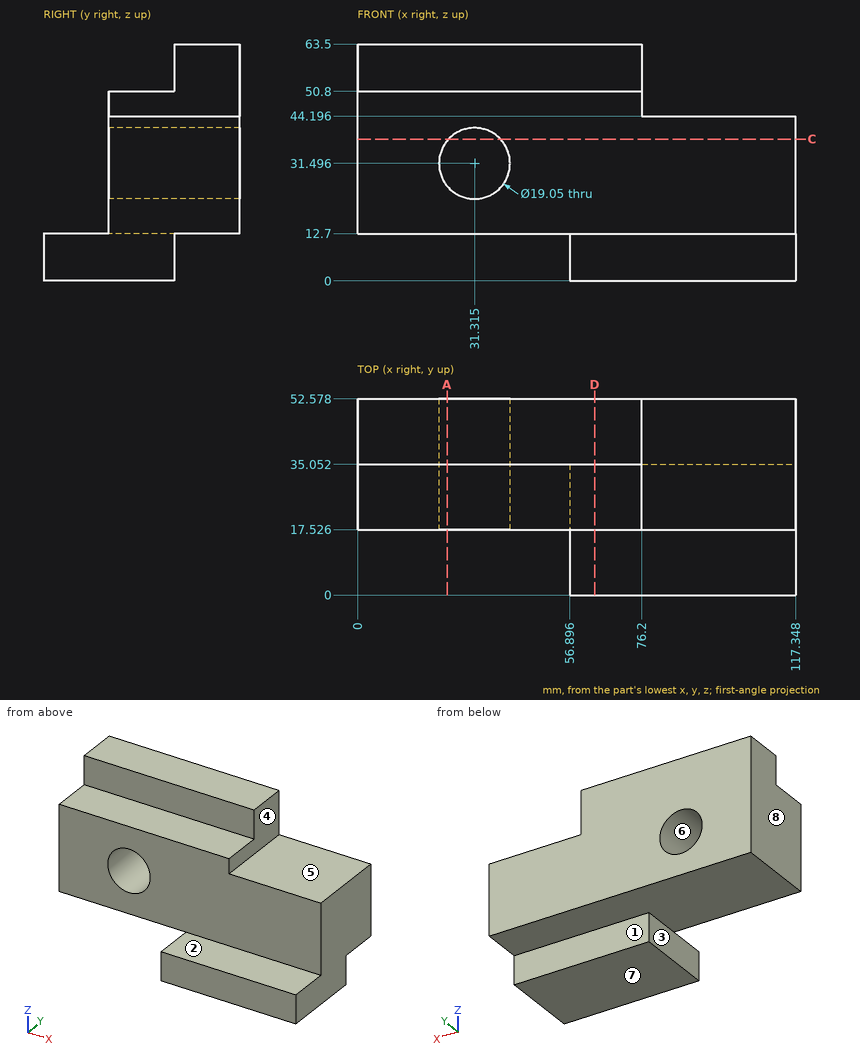
Input: dimensioned drawing with shaded views. Units: mm. Origin: part minimum x, y, z. A direction names the side the tool comes from. Round coordinates to 2 decimals unless told otherwise and drop trailing zeros. Loops run counter-clockwise (first coordinate to the right, second up) from the corner with the lowest first, then second, coordinate; pieces in that order, holes last. Notation, with made-up numbers: (-2.75, -33.5) -> (21.25, -33.5) arc R27 cw to (21.25, 1.5) -> close; hole circle Ø3 at (45.25, 32). An arc over 180 degrees is marked (long way). Answer as a JSON object with one key per item and string values. Group by question number.
1) Reachability of the marked faces 1, 2, 3 and 4 from +Z, -Z, +X, -X, +Y, -Y: full face, straight path, thin tool, end or side. Return the list, or none.
2) Section query D-D on x = 63.5. Output: boundary loops of the cut face in (y, z).
3) Section query A-A on x = 24. Output: boundary loops of the cut face in (y, z).
4) Draft query along Z for the marked faces 5, 6, 7 and 8. Return one class per face: +Z half, -Z half, draft (parallel to the pull), parting line (faces both ways), or undercut.
5) Ray query, L1, parallel to Y at x = 43, z = 58.5; L2, parallel to Z at x = 90.5, y = 27.5; L3, parallel to Z at x = 100, y = 17. Return the intervals inside material, ascending.
6) Section query C-C on z = 38. Output: boundary loops of the cut face in (x, y), plus the area to 3 significant figures.
7) Pin query (flat end, axial travel): pin 1 (4 mm diameter, centred on x = 86.5, z = 4, fed in from +Y); pin 2 (14 mm diameter, centred on y = 24.5, z = 5.5, fed in from -X); pin 3 (1 mm diameter, centred on x = 29, z = 55.5, fed in from -Y); pin 4 (15 mm diameter, centred on x = 31.32, z = 31.5, fed in from -Y). Return the tip coordinate at first contact, or that it passes through.
Reply:
{
 "1": {"face 1": "-Z, +X, -X, +Y", "face 2": "+Z, +X, -X, -Y", "face 3": "-Z, -X, +Y, -Y", "face 4": "+Z, +X, +Y, -Y"},
 "2": {"outline": "(0, 0) -> (35.05, 0) -> (35.05, 12.7) -> (52.58, 12.7) -> (52.58, 63.5) -> (35.05, 63.5) -> (35.05, 50.8) -> (17.53, 50.8) -> (17.53, 12.7) -> (0, 12.7) -> close"},
 "3": {"outline": "(17.53, 12.7) -> (52.58, 12.7) -> (52.58, 25.4) -> (17.53, 25.4) -> close; (17.53, 37.6) -> (52.58, 37.6) -> (52.58, 63.5) -> (35.05, 63.5) -> (35.05, 50.8) -> (17.53, 50.8) -> close"},
 "4": {"face 5": "+Z half", "face 6": "undercut", "face 7": "-Z half", "face 8": "draft"},
 "5": {"L1": "y = 35.05 to 52.58", "L2": "z = 0 to 44.2", "L3": "z = 0 to 12.7"},
 "6": {"outline": "(0, 17.53) -> (24.36, 17.53) -> (24.36, 52.58) -> (0, 52.58) -> close; (38.27, 17.53) -> (117.35, 17.53) -> (117.35, 52.58) -> (38.27, 52.58) -> close", "area": "3,630 mm2"},
 "7": {"pin 1": "stops at y = 35.05", "pin 2": "stops at x = 56.9", "pin 3": "stops at y = 35.05", "pin 4": "passes through"}
}
